from build123d import *

# Parameters (mm, degrees)
F1_DEPTH = 4.7
F3_DEPTH = 1.05
F6_DEPTH = 2
F7_SIZE  = 1


with BuildPart() as f1:
    # F0 (on Front) → F1 (new body)
    with BuildSketch(Plane.XZ):
        with BuildLine():
            Line((0, 31.2), (0, 0))
            Line((0, 0), (19.75, 0))
            Line((19.75, 0), (19.75, 31.2))
            Line((19.75, 31.2), (11.425, 31.2))
            Line((11.425, 31.2), (11.425, 31.4))
            Line((11.425, 31.4), (19.75, 31.4))
            Line((19.75, 31.4), (19.75, 52.5))
            Line((19.75, 52.5), (19.75, 55.1716775767))
            ThreePointArc((19.75, 55.1716775767), (18.375, 59.5), (19.75, 63.8283224233))
            Line((19.75, 63.8283224233), (19.75, 65))
            Line((19.75, 65), (0, 65))
            Line((0, 65), (0, 63.8283224233))
            ThreePointArc((0, 63.8283224233), (1.0229892277, 61.7707377656), (1.375, 59.5))
            ThreePointArc((1.375, 59.5), (1.0229892277, 57.2292622344), (0, 55.1716775767))
            Line((0, 55.1716775767), (0, 52.5))
            Line((0, 52.5), (0, 31.4))
            Line((0, 31.4), (8.325, 31.4))
            Line((8.325, 31.4), (8.325, 31.2))
            Line((8.325, 31.2), (0, 31.2))
        make_face()
        with BuildLine():
            Line((-2, 52.5), (0, 52.5))
            Line((0, 52.5), (0, 55.1716775767))
            ThreePointArc((0, 55.1716775767), (-0.9094386331, 54.1103878035), (-2, 53.2362650918))
            Line((-2, 53.2362650918), (-2, 52.5))
        make_face()
        with BuildLine():
            Line((19.75, 55.1716775767), (19.75, 52.5))
            Line((19.75, 52.5), (21.75, 52.5))
            Line((21.75, 52.5), (21.75, 53.2362650918))
            ThreePointArc((21.75, 53.2362650918), (20.6594386331, 54.1103878035), (19.75, 55.1716775767))
        make_face()
    extrude(amount=F1_DEPTH)

    # F2 (on face) → F3 (cut)
    with BuildSketch(Plane.XZ.offset(4.7)):
        Polygon((13.475, 37.5), (6.275, 37.5), (6.275, 2.2), (6.275, 0), (13.475, 0), (13.475, 2.2), align=None)
    extrude(amount=-F3_DEPTH, mode=Mode.SUBTRACT)

    # F5 (on face) → F6 (join)
    with BuildSketch(Plane.XZ.offset(4.7)):
        with BuildLine():
            Line((-2, 52.5), (0, 52.5))
            Line((0, 52.5), (19.75, 52.5))
            Line((19.75, 52.5), (21.75, 52.5))
            Line((21.75, 52.5), (21.75, 53.2362650918))
            ThreePointArc((21.75, 53.2362650918), (18.5052276407, 58.1084342015), (19.75, 63.8283224233))
            Line((19.75, 63.8283224233), (19.75, 65))
            Line((19.75, 65), (0, 65))
            Line((0, 65), (0, 63.8283224233))
            ThreePointArc((0, 63.8283224233), (1.2447723593, 58.1084342015), (-2, 53.2362650918))
            Line((-2, 53.2362650918), (-2, 52.5))
        make_face()
    extrude(amount=F6_DEPTH)

    # F7
    f7_edges = [f1.edges().sort_by_distance(p)[0] for p in [
        (0, -2.35, 0),
        (19.75, -2.35, 0),
        (3.1375, -4.7, 0),
        (16.6125, -4.7, 0),
        (9.875, -3.65, 0),
    ]]
    chamfer(f7_edges, length=F7_SIZE)


solid = f1.part
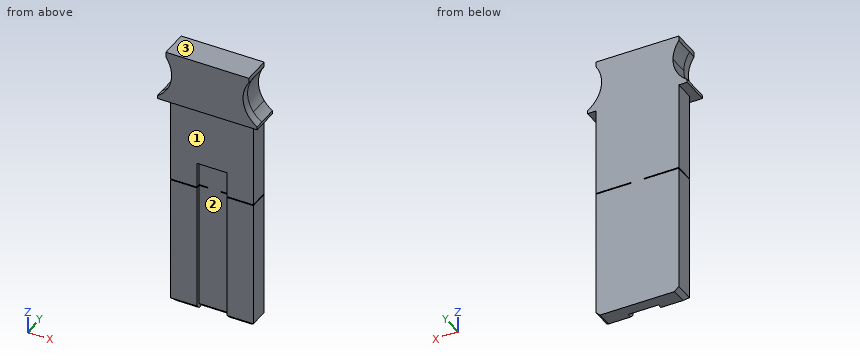
The listing builds one solid part. Answer for the finished solid, in the listing's coordinates (mm). Face numbers are marked on the shaded views. A direction names the side the tool comes from. Give positions to 0.01 mm unless a question says otherwise; leave off trailing zeros. Write each loop counter-clockwise with the first axis right and the second up, starting at its lowest first coordinate (ties: lowest second). Pieces come first, ordered by that corner, then holes.
Item 1: Which of the six approach directions +Z, -Z, +X, -X, +Y, -Y give full straight-line access (tool end or side, diameter ignored) to the marked faces 1, 2 and 3?
Item 2: Section B-B, the plane z = 5 is taken. Write down the section's boundary in (x, y) (3 decimals), plus the area to 3 significant figures.
Item 3: Find the intervals of material crossed by line 1 along X through (y, z) = (-4.25, 20.5) (3 decimals); line 2 along Z through (x, y) = (3.5, -3); line 3 along Z through (x, y) = (19, -0.25), in increasing order.
Item 4: Section C-C, the plane y = -6 is taken. Write down the section's boundary in (x, z) (3 decimals), plus the area to 3 significant figures.
Item 5: Section A-A, the plane x = 15 is taken. Write down the section's boundary in (y, z).
Item 6: Section D-D, the plane x = 9.75 is taken. Write down the section's boundary in (y, z), plus the area to 3 significant figures.
Item 7: Flat-ended cylindrical pins translate along their axes: P1, Ø5, axis at x = 2, z = 14.5, coming from the -Y side; P2, Ø2.5, axis at y = -3, z = 18, coming from the +X side; P3, Ø2.5, axis at y = -2.5, z = 45.5, coming from the -X side. Find the tip coordinate at first contact, or state that the pin passes through.
Completed:
1. face 1: -Z, +X, -X, -Y
1. face 2: -Z, -Y
1. face 3: +Z, +X, -X, +Y, -Y
2. outline: (0, -4.7) - (6.275, -4.7) - (6.275, -3.65) - (13.475, -3.65) - (13.475, -4.7) - (19.75, -4.7) - (19.75, 0) - (0, 0) - close
2. area: 85.3 mm2
3. line 1: x = 0 to 6.275, 13.475 to 19.75
3. line 2: z = 0 to 31.2, 31.4 to 65
3. line 3: z = 0.25 to 31.2, 31.4 to 56.5, 62.5 to 65
4. outline: (-2, 52.5) - (21.75, 52.5) - (21.75, 53.236) arc R7.5 cw to (19.75, 63.828) - (19.75, 65) - (0, 65) - (0, 63.828) arc R7.5 cw to (-2, 53.236) - close
4. area: 237 mm2
5. outline: (-6.7, 52.5) - (-4.7, 52.5) - (-4.7, 31.4) - (0, 31.4) - (0, 65) - (-6.7, 65) - close; (-4.7, 1) - (-3.7, 0) - (0, 0) - (0, 31.2) - (-4.7, 31.2) - close
6. outline: (-6.7, 52.5) - (-4.7, 52.5) - (-4.7, 37.5) - (-3.65, 37.5) - (-3.65, 1) - (-2.65, 0) - (0, 0) - (0, 65) - (-6.7, 65) - close
6. area: 291 mm2
7. P1: stops at y = -4.7
7. P2: stops at x = 19.75
7. P3: stops at x = 0
